Part model, mm, in its own coordinate system. Face numbers are marked on the shaded views. A direction names the side the tool comes from. Give positions to 0.01 mm unless a question says otherwise; leave off trailing zeros. Order: outer loops, then holes, each group sorted by start corner. A loop starts at its lowest first (then second) coordinate and runs counter-clockwise, first axis right, second up. Notation, with made-up numbers: (23.5, 53) -> (29.5, 53) arc R16 ccw to (29.5, 71) -> close; hole circle Ø5 at (74.5, 22.25). An arc over 180 degrees is marked (long way). Write item = value, one per line. Start each with the question number.
(1) Saw through at B-B, the plane y = 67.5. List the corners of the cut face in (x, z).
(2) Saw through at D-D, the plane y = 92.5. List the corners of the cut face in (x, z).
(3) Saw through at A-A, the plane z = -3.75. List the corners of the cut face in (x, y).
(4) Which spindle directions (+Z, -Z, +X, -X, +Y, -Y) get a long thin tool onto all of the face, cutting with end or side? Do the marked faces 4, 5 and 6. Say none if no direction does.
(5) Probe line 1 along Y through (x, z) = (-8, -4.75); line 2 along Y through (x, z) = (0, 2.3); line 3 along Z through (x, y) = (0.25, 80). List the from-to ranges inside material, lowest first. Write a range as from..to.
(6) Flat gauge pins, fed straight in: pin 1 (3 mm diameter, centred on x = -5, y = 69, fed in from +Z); pin 2 (1.5 mm diameter, centred on y = 40, z = -1.5, fed in from -X); pin 3 (5 mm diameter, centred on x = 2.5, z = -5, fed in from +Y). Where does each tip first touch, or does it go through?
(7) Two-plate mould, pull along Y, no slides. Class the marked faces 1, 2 and 3: pulls with the +Y half, pulls with the -Y half, needs draft (parallel to the pull), parting line crosses it, or undercut.
(8) Saw through at C-C, the plane y = 21. List the corners of the cut face in (x, z), then the cut area to 3 significant figures.
from build123d import *

# Parameters (mm, degrees)
SKETCH1_R           = 10
BOSS_EXTRUDE1_DEPTH = 100
SKETCH4_W           = 20
SKETCH4_H           = 25
CUT_EXTRUDE2_DEPTH  = 10
SKETCH7_R           = 5
BOSS_EXTRUDE2_DEPTH = 5
FILLET7_R           = 5
SKETCH9_R           = 5
CUT_EXTRUDE3_DEPTH  = 5
FILLET8_R           = 5


with BuildPart() as part:
    # Sketch1 → Boss-Extrude1 (new body)
    with BuildSketch(Plane(origin=(0, 0, 0), x_dir=(1, 0, 0), z_dir=(0, 1, 0))):
        with Locations(Location((0, 0, 0), (0, 0, 90))):
            Circle(SKETCH1_R)
    extrude(amount=BOSS_EXTRUDE1_DEPTH)

    # Sketch4 → Cut-Extrude2 (cut)
    with BuildSketch(Plane.XY):
        with Locations((0, 87.5)):
            Rectangle(SKETCH4_W, SKETCH4_H)
    cut_extrude2 = extrude(amount=-CUT_EXTRUDE2_DEPTH, mode=Mode.SUBTRACT)

    # Sketch7 → Boss-Extrude2 (add)
    with BuildSketch(Plane.XY):
        with Locations((0, 90.066469536)):
            Circle(SKETCH7_R)
        with Locations((0, 9.933530464)):
            Circle(SKETCH7_R)
    extrude(amount=-BOSS_EXTRUDE2_DEPTH)

    # Fillet7
    # the kernel refuses this fillet: 5 mm, written as the material it takes off along each edge
    with BuildSketch(Plane(origin=(-22.5, 100, 0), x_dir=(0, -1, 0), z_dir=(1, 0, 0))) as fillet7_piece_1_section:
        with BuildLine():
            CenterArc((FILLET7_R, -FILLET7_R), FILLET7_R, 90, 90)
            Line((0, -FILLET7_R), (0, 0))
            Line((0, 0), (FILLET7_R, 0))
        make_face()
    fillet7_piece_1 = extrude(amount=45, mode=Mode.PRIVATE)
    fillet7_piece_1 = fillet7_piece_1 - Plane(origin=(0, 90.066469536, 1.132005312), x_dir=(1, 0, 0), z_dir=(0, 0, 1)) * Cylinder(5, 110, mode=Mode.PRIVATE)
    add(fillet7_piece_1, mode=Mode.SUBTRACT)
    with BuildSketch(Plane(origin=(0, 100, 0), x_dir=(-0.3134140431814407, 0, -0.9496165739584909), z_dir=(0.9496165739584909, 0, -0.3134140431814407))) as fillet7_piece_2:
        with BuildLine():
            CenterArc((10 - FILLET7_R, -FILLET7_R), FILLET7_R, 0, 90)
            Line((10 - FILLET7_R, 0), (10, 0))
            Line((10, 0), (10, -FILLET7_R))
        make_face()
    revolve(axis=Axis((0, 100, 0), (0, 1, 0)), revolution_arc=323.469804901, mode=Mode.SUBTRACT)

    # Mirror3: Cut-Extrude2 across plane
    add(cut_extrude2.mirror(Plane.ZX.offset(50)), mode=Mode.SUBTRACT)

    # Sketch9 → Cut-Extrude3 (cut)
    with BuildSketch(Plane.XY):
        with Locations((0, 9.933530464)):
            Circle(SKETCH9_R)
    extrude(amount=CUT_EXTRUDE3_DEPTH, mode=Mode.SUBTRACT)

    # Fillet8
    # the kernel refuses this fillet: 5 mm, written as the material it takes off along each edge
    with BuildSketch(Plane(origin=(0, 0, 0), x_dir=(-0.31341404318144095, 0, -0.9496165739584909), z_dir=(0.9496165739584909, 0, -0.31341404318144095))) as fillet8_piece_1:
        with BuildLine():
            CenterArc((10 - FILLET8_R, FILLET8_R), FILLET8_R, 270, 90)
            Line((10 - FILLET8_R, 0), (10, 0))
            Line((10, 0), (10, FILLET8_R))
        make_face()
    revolve(axis=Axis((0, 0, 0), (0, 1, 0)), revolution_arc=323.469804901, mode=Mode.SUBTRACT)
    with BuildSketch(Plane(origin=(-22.5, 0, 0), x_dir=(0, 0, 1), z_dir=(1, 0, 0))) as fillet8_piece_2:
        with BuildLine():
            CenterArc((FILLET8_R, -FILLET8_R), FILLET8_R, 90, 90)
            Line((0, -FILLET8_R), (0, 0))
            Line((0, 0), (FILLET8_R, 0))
        make_face()
    extrude(amount=45, mode=Mode.SUBTRACT)


solid = part.part
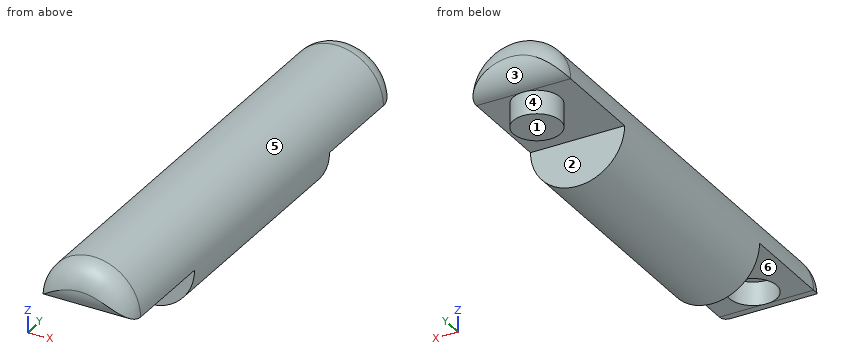
Results list:
q1.outline = circle Ø20 at (0, 0)
q2.outline = (-10, 0) -> (-4.37, 0) -> (-4.37, -5) -> (4.37, -5) -> (4.37, 0) -> (10, 0) arc R10 ccw to start
q3.outline = (-9.27, 25) -> (9.27, 25) -> (9.27, 75) -> (-9.27, 75) -> close; circle Ø10 at (0, 90.07)
q4.face_4 = -Z
q4.face_5 = +Y, -Y
q4.face_6 = -Z, +X, -X, -Y
q5.line_1 = 25..75
q5.line_2 = 0.79..4.93, 14.93..99.21
q5.line_3 = 0..10
q6.pin_1 = 9.37
q6.pin_2 = -9.97
q6.pin_3 = 95.07
q7.face_1 = needs draft
q7.face_2 = undercut
q7.face_3 = pulls with the +Y half
q8.outline = (-10, 0) -> (10, 0) arc R10 ccw to start
q8.area = 157 mm^2
